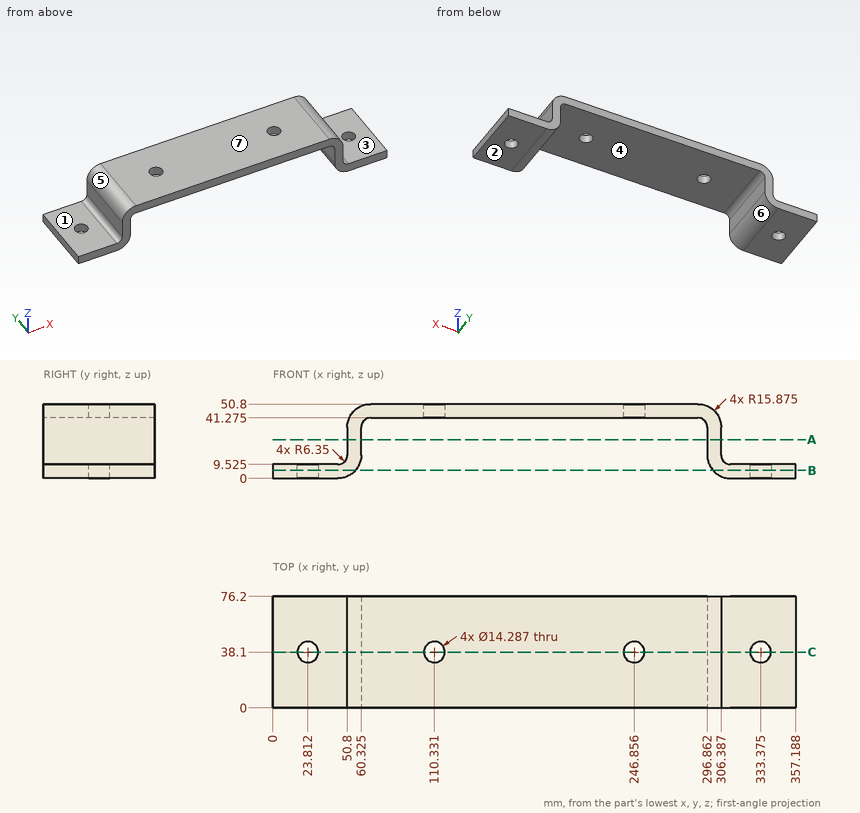
Study the drawing (mm; zero at the part's minimum x, y, z) and answer. A direction names the side the tool comes from. Give positions to 0.01 mm unless a question says otherwise; leave off trailing zeros. Order: outer loops, then holes, each group sorted by start corner. A loop starts at its lowest first (then second) coordinate and runs counter-clockwise, first axis right, second up. Notation, with made-up numbers: (-30.75, -5.5) - (22.25, -5.5) arc R20 cw to (22.25, 2.5) - close; hole circle Ø3 at (-6.75, -21). An arc over 180 degrees is marked (long way). Answer in a Markdown table with one row per item. Add a question column.
Q1. The part is cut by section C-C (y = 38.1). Give the number of separate pieces and of enclosed holes in the cut face, then the cut area to 3 significant figures.
Q2. Which of the six approach directions +Z, -Z, +X, -X, +Y, -Y give full straight-line access (tool end or side, diameter ignored) to the marked faces 1, 2, 3 and 4?
Q3. For a pull along X with two mould halves and no side action, classify the marked faces 5, 6 and 7 as released by +X, released by -X, zero draft, split by the parting line, or undercut.
Q4. Given P1, Ø23, axis at x = 143, y = 33, coming from the -Z side (1 decimal); P2, Ø5, axis at y = 50, z = 22, coming from the -X side; P3, Ø22, axis at x = 29, y = 53.5, coming from the +Z side (1 decimal), each flat-ended and moving along its own axis, determine where each tip first touches the part or whether it passes through.
Q5. The part is cut by section A-A (z = 26.5). Determine the outline of the cut face in (x, y) (1 decimal).
Q6. The part is cut by section B-B (z = 5.5). Determine the outline of the cut face in (x, y) (1 decimal).
Q7. Find the intervals of material crossed by line 1 along Z through (x, y) = (182, 23) (1 decimal); line 2 along Z through (x, y) = (340.5, 48.5) (1 decimal); line 3 along X through (y, z) = (68, 4) (1 decimal), in increasing order. Write a range as [from, to].
Determined:
| question | item | result |
|---|---|---|
| 1 | separate pieces | 5 |
| 1 | enclosed holes | 0 |
| 1 | area | 3,460 mm² |
| 2 | face 1 | +Z, -X, +Y, -Y |
| 2 | face 2 | -Z, +X, -X, +Y, -Y |
| 2 | face 3 | +Z, +X, +Y, -Y |
| 2 | face 4 | -Z, +Y, -Y |
| 3 | face 5 | released by -X |
| 3 | face 6 | undercut |
| 3 | face 7 | zero draft |
| 4 | P1 | stops at z = 41.3 |
| 4 | P2 | stops at x = 50.8 |
| 4 | P3 | stops at z = 9.5 |
| 5 | outline | (50.8, 0) - (60.3, 0) - (60.3, 76.2) - (50.8, 76.2) - close; (296.9, 0) - (306.4, 0) - (306.4, 76.2) - (296.9, 76.2) - close |
| 6 | outline | (0, 0) - (56.5, 0) - (56.5, 76.2) - (0, 76.2) - close; (300.7, 0) - (357.2, 0) - (357.2, 76.2) - (300.7, 76.2) - close; hole circle Ø14.3 at (23.8, 38.1); hole circle Ø14.3 at (333.4, 38.1) |
| 7 | line 1 | z = [41.3, 50.8] |
| 7 | line 2 | z = [0, 9.5] |
| 7 | line 3 | x = [0, 55], [302.2, 357.2] |
